Read the model definition and answer for the solid it produces. Units are mm, in the model's axes. A direction names the side the tool comes from. Give positions to 0.01 mm unless a question says otherwise; leave off trailing zeros. Loops run counter-clockwise (first coordinate to the right, second up) from the corner with the lowest first, then second, coordinate; pieces in that order, holes last. Notation, with made-up numbers: (-12, -28) - (-1, -28) arc R24 cw to (-1, -9) - close; hole circle Ø8 at (43.5, 18). An arc over 180 degrees is marked (long way). Put each result on its own line as item: value. Start each with the question number.
1. For a pull along Z with two mould halves and no side action, classify faces 6 (the cylindrical face through (-0.647, -79.994, 7.395)), 7 (the flat face through (-1, 19, -327)) as released by +Z, released by -Z, zero draft, split by the parting line, or undercut.
2. A cutting plane is placed at A-A, the plane z = -129. Determine the outline of the cut face in (x, y).
3. A cutting plane is placed at B-B, the plane z = 39. Determine the outline of the cut face in (x, y).
4. Consider L1, parallel to Z at x = -42, y = -55.5; L2, parallel to Z at x = 41, y = 48.5; L3, parallel to Z at x = -60.5, y = 3. Determine where each line is inside the solid, lowest interval first. Write a range as from..to.
5. Given pin 1 Ø16 at (x, y) = (-55, 0) entering from +Z; pin 2 Ø1 at (x, z) = (15, 115) entering from +Y; pin 3 Ø5 at (y, z) = (-7, -119.5) entering from +X, each flat-ended and moving along its own axis, determine where each tip first touches the part or whether it passes through.
6. For faces 1 (the flat face through (-1, -37, -38)), 2 (the cylindrical face through (-0.647, -79.994, 68.605)), 3 (the cylindrical face through (4.686, 35.694, 94.734)), 4 (the cylindrical face through (-40.81, 43.51, -387.4)), 5 (the flat face through (49.333, 4.207, -45.395)), determine the directions among +Z, -Z, +X, -X, +Y, -Y from which every point of the face is accessible in a straight line to the end or side of a thin tool.
```python
from build123d import *

# Parameters (mm, degrees)
SKETCH1_R             = 36
BOSS_EXTRUDE1_DEPTH   = 15
SKETCH2_R             = 27
BOSS_EXTRUDE2_DEPTH   = 46
SKETCH3_R             = 36
BOSS_EXTRUDE3_DEPTH   = 38
BODY_MOVE_COPY1_ANGLE = 180
SKETCH4_R             = 17.5
BOSS_EXTRUDE4_DEPTH   = 80
SKETCH5_R             = 72
SKETCH5_R_2           = 5
BOSS_EXTRUDE5_DEPTH   = 15


with BuildPart() as part:
    # Sketch1 → Boss-Extrude1 (new body)
    with BuildSketch(Plane.XY):
        with BuildLine():
            ThreePointArc((64.569893475, 47.23059238), (0, 80), (-64.569893475, 47.23059238))
            Line((-64.569893475, 47.23059238), (-34.517510455, -54.224552409))
            ThreePointArc((-34.517510455, -54.224552409), (-5.165734392, -8.372550074), (36, -44))
            ThreePointArc((36, -44), (35.627449926, -49.165734392), (34.517510455, -54.224552409))
            Line((34.517510455, -54.224552409), (64.569893475, 47.23059238))
        make_face()
        with Locations((0, -44)):
            Circle(SKETCH1_R)
    boss_extrude1 = extrude(amount=BOSS_EXTRUDE1_DEPTH)

    # Sketch2 → Boss-Extrude2 (add)
    with BuildSketch(Plane.XY.offset(15)):
        with Locations((0, -44)):
            Circle(SKETCH2_R)
    extrude(amount=BOSS_EXTRUDE2_DEPTH)

    # Sketch3 → Boss-Extrude3 (add)
    with BuildSketch(Plane(origin=(0, 0, 0), x_dir=(-1, 0, 0), z_dir=(0, 0, -1))):
        Circle(SKETCH3_R)
    boss_extrude3 = extrude(amount=BOSS_EXTRUDE3_DEPTH)

    # Mirror1: Boss-Extrude1, Boss-Extrude3 across plane
    add(boss_extrude1.mirror(Plane.XY.offset(38)))
    add(boss_extrude3.mirror(Plane.XY.offset(38)))


with BuildPart() as body_2:
    # Mirror6: mirrored copy
    add(part.part.mirror(Plane(origin=(0, 0, -19), x_dir=(1, 0, 0), z_dir=(0, 0, -1))))


with BuildPart() as body_2_1:
    # Body-Move/Copy1: moved
    add(body_2.part.rotate(Axis((0, 0, -76), (1, 0, 0)), BODY_MOVE_COPY1_ANGLE))


with BuildPart() as body_3:
    # Mirror7: mirrored copy
    add(body_2_1.part.mirror(Plane(origin=(0, 0, -133), x_dir=(1, 0, 0), z_dir=(0, 0, -1))))


with BuildPart() as body_4:
    # Mirror7 2: mirrored copy
    add(part.part.mirror(Plane(origin=(0, 0, -133), x_dir=(1, 0, 0), z_dir=(0, 0, -1))))

    # Sketch5 → Boss-Extrude5 (add)
    with BuildSketch(Plane(origin=(0, 0, -380), x_dir=(-1, 0, 0), z_dir=(0, 0, -1))):
        with Locations(Location((0, 0, 0), (0, 0, 90))):
            Circle(SKETCH5_R)
        with Locations(Location((0, 55, 0), (0, 0, 90))):
            Circle(SKETCH5_R_2, mode=Mode.SUBTRACT)
        with Locations(Location((38.890872965, 38.890872965, 0), (0, 0, 90))):
            Circle(SKETCH5_R_2, mode=Mode.SUBTRACT)
        with Locations(Location((55, 0, 0), (0, 0, 90))):
            Circle(SKETCH5_R_2, mode=Mode.SUBTRACT)
        with Locations(Location((38.890872965, -38.890872965, 0), (0, 0, 90))):
            Circle(SKETCH5_R_2, mode=Mode.SUBTRACT)
        with Locations(Location((0, -55, 0), (0, 0, 90))):
            Circle(SKETCH5_R_2, mode=Mode.SUBTRACT)
        with Locations(Location((-38.890872965, -38.890872965, 0), (0, 0, 90))):
            Circle(SKETCH5_R_2, mode=Mode.SUBTRACT)
        with Locations(Location((-55, 0, 0), (0, 0, 90))):
            Circle(SKETCH5_R_2, mode=Mode.SUBTRACT)
        with Locations(Location((-38.890872965, 38.890872965, 0), (0, 0, 90))):
            Circle(SKETCH5_R_2, mode=Mode.SUBTRACT)
    extrude(amount=BOSS_EXTRUDE5_DEPTH)


with BuildPart() as part_1:
    add(part.part)

    # Sketch4 → Boss-Extrude4 (add)
    with BuildSketch(Plane.XY.offset(114)):
        Circle(SKETCH4_R)
    extrude(amount=BOSS_EXTRUDE4_DEPTH)

    # Combine1: union body 2, body 3, body 4
    add(body_2_1.part)
    add(body_3.part)
    add(body_4.part)


solid = part_1.part
```
Return value:
1. face 6: zero draft
1. face 7: undercut
2. outline: circle Ø72 at (0, 0)
3. outline: circle Ø54 at (0, -44)
4. L1: z = -395..-380, -228..-213, -167..-152, -114..-99, -53..-38
4. L2: z = -395..-380, -342..-327, -281..-266, 0..15, 61..76
4. L3: z = -395..-380
5. pin 1: stops at z = 76
5. pin 2: stops at y = 9.8
5. pin 3: stops at x = 35.72
6. face 1: none
6. face 2: +Z, -Y
6. face 3: +Z
6. face 4: -Z
6. face 5: +X, +Y
